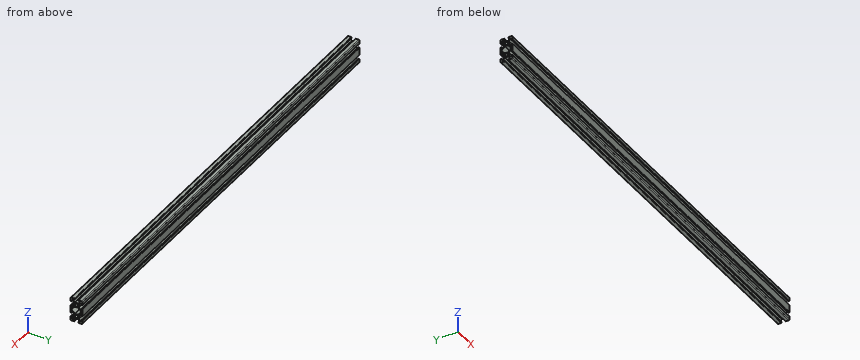
from build123d import *

# Parameters (mm, degrees)
SKETCH1_R                = 2.5
F_20_X_40_X_T1_5_1_DEPTH = 760


with BuildPart() as part:
    # Sketch1 → 铝型材 20 X 40 X T1.5(1) (new body)
    with BuildSketch(Plane.YZ):
        with BuildLine():
            Line((-3.6, 10), (-3.6, 9.5))
            Line((-3.6, 9.5), (-3.1, 9.5))
            Line((-3.1, 9.5), (-3.1, 8.5))
            Line((-3.1, 8.5), (-5.5, 8.5))
            Line((-5.5, 8.5), (-5.5, 6.65))
            Line((-5.5, 6.65), (-2.75, 3.9))
            Line((-2.75, 3.9), (2.75, 3.9))
            Line((2.75, 3.9), (5.5, 6.65))
            Line((5.5, 6.65), (5.5, 8.5))
            Line((5.5, 8.5), (3.1, 8.5))
            Line((3.1, 8.5), (3.1, 9.5))
            Line((3.1, 9.5), (3.6, 9.5))
            Line((3.6, 9.5), (3.6, 10))
            Line((3.6, 10), (8.5, 10))
            ThreePointArc((8.5, 10), (9.560660172, 9.560660172), (10, 8.5))
            Line((10, 8.5), (10, 3.6))
            Line((10, 3.6), (9.5, 3.6))
            Line((9.5, 3.6), (9.5, 3.1))
            Line((9.5, 3.1), (8.5, 3.1))
            Line((8.5, 3.1), (8.5, 5.5))
            Line((8.5, 5.5), (6.65, 5.5))
            Line((6.65, 5.5), (3.9, 2.75))
            Line((3.9, 2.75), (3.9, -2.75))
            Line((3.9, -2.75), (6.65, -5.5))
            Line((6.65, -5.5), (8.5, -5.5))
            Line((8.5, -5.5), (8.5, -3.1))
            Line((8.5, -3.1), (9.5, -3.1))
            Line((9.5, -3.1), (9.5, -3.6))
            Line((9.5, -3.6), (10, -3.6))
            Line((10, -3.6), (10, -16.4))
            Line((10, -16.4), (9.5, -16.4))
            Line((9.5, -16.4), (9.5, -16.9))
            Line((9.5, -16.9), (8.5, -16.9))
            Line((8.5, -16.9), (8.5, -14.5))
            Line((8.5, -14.5), (6.65, -14.5))
            Line((6.65, -14.5), (3.9, -17.25))
            Line((3.9, -17.25), (3.9, -22.75))
            Line((3.9, -22.75), (6.65, -25.5))
            Line((6.65, -25.5), (8.5, -25.5))
            Line((8.5, -25.5), (8.5, -23.1))
            Line((8.5, -23.1), (9.5, -23.1))
            Line((9.5, -23.1), (9.5, -23.6))
            Line((9.5, -23.6), (10, -23.6))
            Line((10, -23.6), (10, -28.5))
            ThreePointArc((10, -28.5), (9.560660172, -29.560660172), (8.5, -30))
            Line((8.5, -30), (3.6, -30))
            Line((3.6, -30), (3.6, -29.5))
            Line((3.6, -29.5), (3.1, -29.5))
            Line((3.1, -29.5), (3.1, -28.5))
            Line((3.1, -28.5), (5.5, -28.5))
            Line((5.5, -28.5), (5.5, -26.65))
            Line((5.5, -26.65), (2.75, -23.9))
            Line((2.75, -23.9), (-2.75, -23.9))
            Line((-2.75, -23.9), (-5.5, -26.65))
            Line((-5.5, -26.65), (-5.5, -28.5))
            Line((-5.5, -28.5), (-3.1, -28.5))
            Line((-3.1, -28.5), (-3.1, -29.5))
            Line((-3.1, -29.5), (-3.6, -29.5))
            Line((-3.6, -29.5), (-3.6, -30))
            Line((-3.6, -30), (-8.5, -30))
            ThreePointArc((-8.5, -30), (-9.560660172, -29.560660172), (-10, -28.5))
            Line((-10, -28.5), (-10, -23.6))
            Line((-10, -23.6), (-9.5, -23.6))
            Line((-9.5, -23.6), (-9.5, -23.1))
            Line((-9.5, -23.1), (-8.5, -23.1))
            Line((-8.5, -23.1), (-8.5, -25.5))
            Line((-8.5, -25.5), (-6.65, -25.5))
            Line((-6.65, -25.5), (-3.9, -22.75))
            Line((-3.9, -22.75), (-3.9, -17.25))
            Line((-3.9, -17.25), (-6.65, -14.5))
            Line((-6.65, -14.5), (-8.5, -14.5))
            Line((-8.5, -14.5), (-8.5, -16.9))
            Line((-8.5, -16.9), (-9.5, -16.9))
            Line((-9.5, -16.9), (-9.5, -16.4))
            Line((-9.5, -16.4), (-10, -16.4))
            Line((-10, -16.4), (-10, -3.6))
            Line((-10, -3.6), (-9.5, -3.6))
            Line((-9.5, -3.6), (-9.5, -3.1))
            Line((-9.5, -3.1), (-8.5, -3.1))
            Line((-8.5, -3.1), (-8.5, -5.5))
            Line((-8.5, -5.5), (-6.65, -5.5))
            Line((-6.65, -5.5), (-3.9, -2.75))
            Line((-3.9, -2.75), (-3.9, 2.75))
            Line((-3.9, 2.75), (-6.65, 5.5))
            Line((-6.65, 5.5), (-8.5, 5.5))
            Line((-8.5, 5.5), (-8.5, 3.1))
            Line((-8.5, 3.1), (-9.5, 3.1))
            Line((-9.5, 3.1), (-9.5, 3.6))
            Line((-9.5, 3.6), (-10, 3.6))
            Line((-10, 3.6), (-10, 8.5))
            ThreePointArc((-10, 8.5), (-9.560660172, 9.560660172), (-8.5, 10))
            Line((-8.5, 10), (-3.6, 10))
        make_face()
        Circle(SKETCH1_R, mode=Mode.SUBTRACT)
        with Locations((0, -20)):
            Circle(SKETCH1_R, mode=Mode.SUBTRACT)
        Polygon((8.85, -10), (2.75, -3.9), (-2.75, -3.9), (-8.85, -10), (-2.75, -16.1), (2.75, -16.1), align=None, mode=Mode.SUBTRACT)
    extrude(amount=F_20_X_40_X_T1_5_1_DEPTH)


solid = part.part
Build history of the part. All positions in model axes, mm. Round coordinates to 2 decimals unless told otherwise and drop trailing zeros. Use CSV: the item, a comma, the result in double quotes.
1. Flat gauge pins, fed straight in: pin 1 (0.6 mm diameter, centred on x = 333, z = -3.5, fed in from -Y); pin 2 (6 mm diameter, centred on x = 324, y = -0.5, fed in from -Z). Where does each tip first touch, or does it go through?
Reply:
pin 1,"stops at y = -10"
pin 2,"stops at z = -29.5"
2. Saw through at A-A (x = 390.5). State how many separate pieces and enclosed holes the cut face has, plus the area to 3 significant figures.
Reply:
separate pieces,"1"
enclosed holes,"3"
area,"300 mm²"
3. Wall check: probe 1 along Z at (x, y) = (335, 4.25); probe 2 along Z at (x, y) = (221, 0); probe 3 along Z at (x, y) = (201, -3.5). Give the ranges that are in metal, low to high. Write a range as from..to.
Reply:
probe 1,"z = -30..-28.5, -25.4..-23.1, -16.9..-14.6, -5.4..-3.1, 3.1..5.4, 8.5..10"
probe 2,"z = -23.9..-22.5, -17.5..-16.1, -3.9..-2.5, 2.5..3.9"
probe 3,"z = -29.5..-28.5, -24.65..-15.35, -4.65..4.65, 8.5..9.5"
